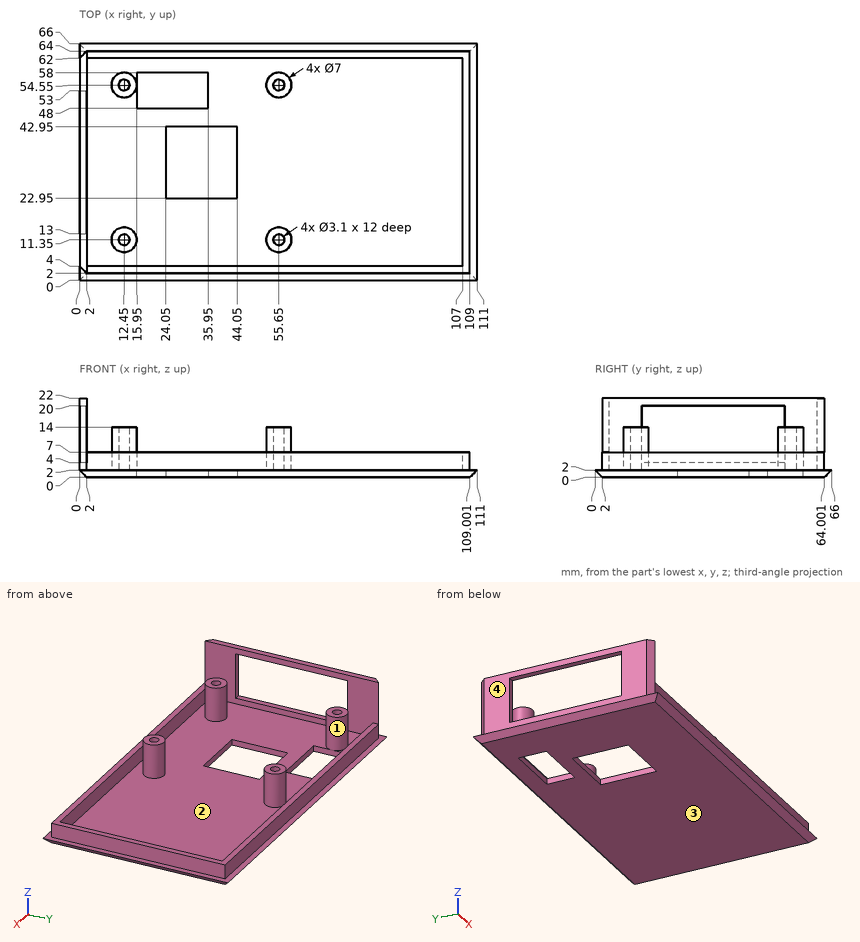
Geometry: see drawing. Coordinates: mm, zero at the bounding-box minimum. Coordinates: 2 decimals unless noted, no trailing zeros. Put each result on its own line as item: value. Start each with the question number.
1) Pull-direction query (X, two-part tool) for the marked faces 1, 2, 3 and 4; classes: pulls with the +X half, pulls with the -X half, needs draft (parallel to the pull), parting line crosses it, or undercut.
2) Ray query, L1, parallel to X at y = 11.35, z = 4.5; L2, parallel to Y at x = 55.65, z = 9; L3, parallel to X at y = 54.55, z = 9.5. Return the intervals inside material, ascending. Write a range as from..to.
3) Contact query for flat-ended pins moving along their axis: pin 1 Ø2 at (x, y) = (13.5, 55) entering from +Z; pin 2 Ø20 at (x, y) = (48.5, 42.5) entering from +Z; pin 3 Ø4 at (x, z) = (34.5, 5.5) entering from +Y. Output: stop coordinate, or through.
The answers:
1. face 1: undercut
1. face 2: undercut
1. face 3: needs draft
1. face 4: pulls with the -X half
2. L1: x = 0..2, 8.95..10.9, 14..15.95, 52.15..54.1, 57.2..59.15, 107..109
2. L2: y = 7.85..9.8, 12.9..14.85, 51.05..53, 56.1..58.05
2. L3: x = 0..2, 8.95..10.9, 14..15.95, 52.15..54.1, 57.2..59.15
3. pin 1: stops at z = 14
3. pin 2: stops at z = 2
3. pin 3: stops at y = 64
